from build123d import *

# Parameters (mm, degrees)
F0_W     = 59.2
F0_H     = 107
F1_DEPTH = 6
F2_W     = 57.2188
F2_H     = 105.0188
F3_DEPTH = 5


with BuildPart() as f1:
    # F0 (on Top) → F1 (new body)
    with BuildSketch(Plane.XY):
        with Locations((-29.6, -1.328537)):
            Rectangle(F0_W, F0_H)
    extrude(amount=F1_DEPTH)

    # F2 (on face) → F3 (cut)
    with BuildSketch(Plane.XY.offset(6)):
        with Locations((-29.6, -1.328537)):
            Rectangle(F2_W, F2_H)
    extrude(amount=-F3_DEPTH, mode=Mode.SUBTRACT)


solid = f1.part
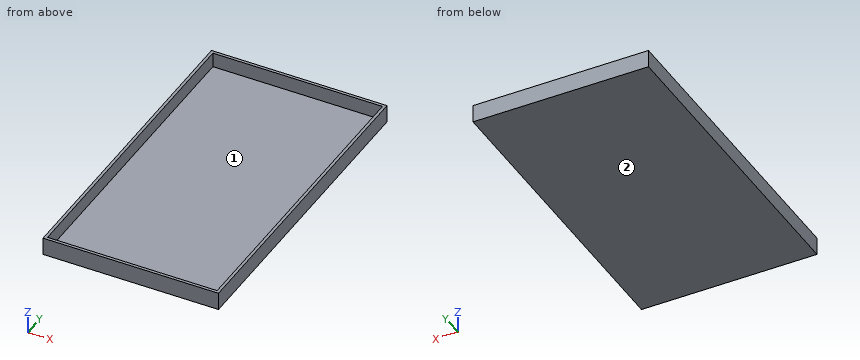
Design review of the part built by this model. Coordinates are the model's own, in mm. Face numbers are marked on the shaded views. Round coordinates to 2 decimals unless told otherwise and drop trailing zeros. Loops run counter-clockwise (first coordinate to the right, second up) from the corner with the lowest first, then second, coordinate; pieces in that order, holes last. Notation, with made-up numbers: M 46.25,-12.75 L 54.25,-12.75 A7 ccw 54.25,-4.75 Z; hole C 17.5,49 d9. An arc over 180 degrees is marked long. Answer as a JSON object with one key per item and string values.
Item 1: Wall thickness on L1, parallel to Y at x = -15.5, z = 5.6; L2, parallel to X at y = -35.5, z = 3.45; L3, parallel to Z at x = -40.5, y = 29: over which ranges is each line inside the solid? List them lowest first. Write a range as from..to.
Answer sheet:
{"L1": "y = -54.83..-53.84, 51.18..52.17", "L2": "x = -59.2..-58.21, -0.99..0", "L3": "z = 0..1"}
Item 2: The part is to be moulded in two halves that separate along Y. For the marked faces 1 and 2, say which applies: pulls with the +Y half, pulls with the -Y half, needs draft (parallel to the pull), parting line crosses it, or undercut.
Answer sheet:
{"face 1": "undercut", "face 2": "needs draft"}
Item 3: We need section B-B on x = -7. Give the boundary of the cut face in (y, z), and give its area (3 significant figures).
Answer sheet:
{"outline": "M -54.83,0 L 52.17,0 L 52.17,6 L 51.18,6 L 51.18,1 L -53.84,1 L -53.84,6 L -54.83,6 Z", "area": "117 mm^2"}
Item 4: We need section C-C on y = 46.5. Give the boundary of the cut face in (x, z).
Answer sheet:
{"outline": "M -59.2,0 L 0,0 L 0,6 L -0.99,6 L -0.99,1 L -58.21,1 L -58.21,6 L -59.2,6 Z"}
Item 5: We need section A-A on z = 3.05. Give the boundary of the cut face in (x, y).
Answer sheet:
{"outline": "M -59.2,-54.83 L 0,-54.83 L 0,52.17 L -59.2,52.17 Z; hole M -58.21,-53.84 L -0.99,-53.84 L -0.99,51.18 L -58.21,51.18 Z"}
Item 6: Clearance check with a flat-ended pin moving along its axis: P1, Ø12, axis at x = -10.5, y = -27.5, coming from the +Z side. State where the tip first meets the part, or that it passes through.
Answer sheet:
{"P1": "stops at z = 1"}
